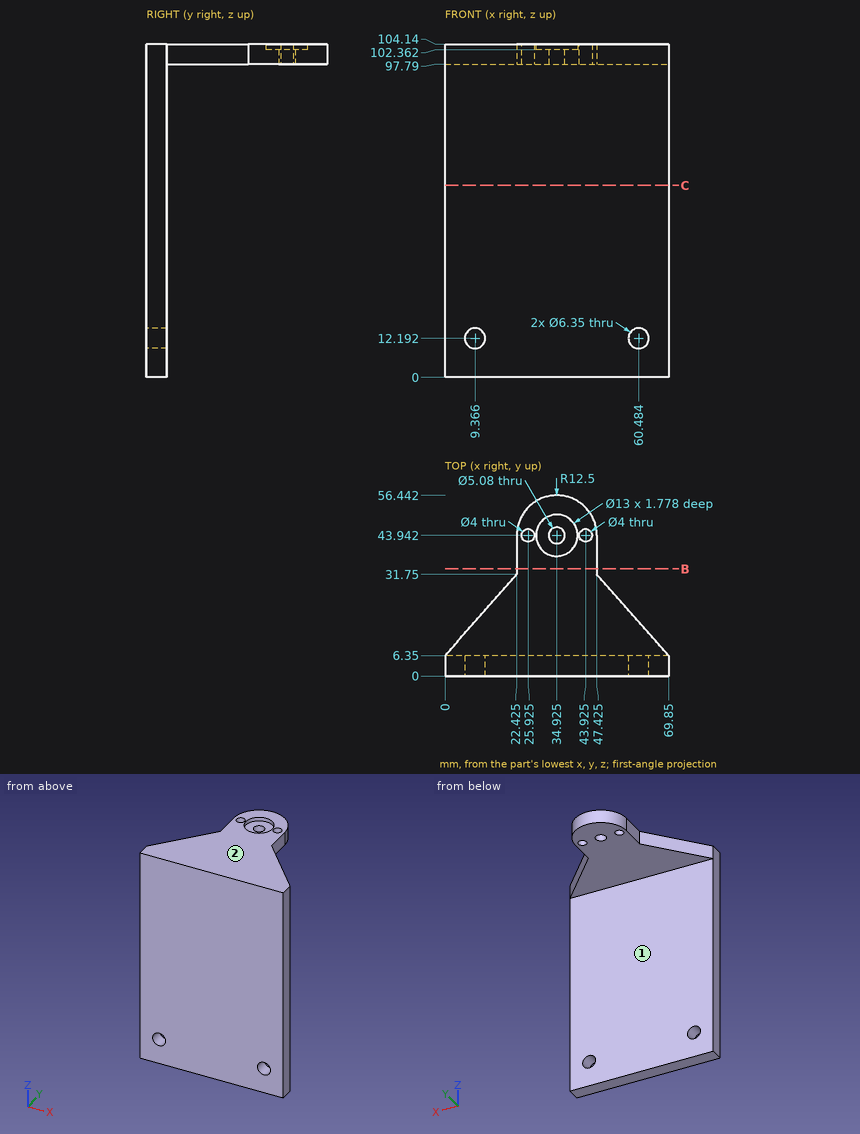
Drawing for the job (mm, zero at the part's lowest x, y, z). A direction names the side the tool comes from. Give positions to 0.01 mm unless a question says otherwise; leave off trailing zeros. Order: outer loops, then holes, each group sorted by start corner. A loop starts at its lowest first (then second) coordinate and runs counter-clockwise, first axis right, second up. Notation, with made-up numbers: M 38,83.5 L 94,83.5 A19 cw 94,95.5 Z; hole C 39.5,77.25 d8. An arc over 180 degrees is marked long. Put each result on its own line as item: value.
Item 1: 3-axis set-ups, long thin cutter, end or side, ignore diameter. For the marked faces 1 and 2: which of +Z, -Z, +X, -X, +Y, -Y reach the whole face in a straight line?
From the geometry:
face 1: -Z, +X, -X, +Y
face 2: +Z, +X, -X, +Y, -Y
Item 2: Flat gauge pins, fed straight in: pin 1 Ø5 at (x, z) = (27.5, 69) entering from +Y; pin 2 Ø15 at (x, y) = (28, 26) entering from -Z; pin 3 Ø3 at (x, y) = (25.925, 43.942) entering from +Z; pin 4 Ø3 at (y, z) = (38.5, 100.5) entering from +X (3 decimals). Where does each tip first touch, or does it go through?
From the geometry:
pin 1: stops at y = 6.35
pin 2: stops at z = 97.79
pin 3: passes through
pin 4: stops at x = 47.425
Item 3: Slice it at C-C, the plane z = 60. Write the cut outline in (x, y).
From the geometry:
outline: M 0,0 L 69.85,0 L 69.85,6.35 L 0,6.35 Z
Item 4: Slice it at B-B, the plane y = 33.5. Write the cut outline in (x, z) (3 decimals), plus the area to 3 significant figures.
From the geometry:
outline: M 22.425,97.79 L 47.425,97.79 L 47.425,104.14 L 22.425,104.14 Z
area: 159 mm2
Item 5: Probe line 1 (Y direction, x = 23, z = 82.5); line 2 (Y direction, x = 36, z = 98) (1 decimal); line 3 (Z direction, x = 8.5, y = 14). List the from-to ranges inside material, lowest first. Write a range as [from, to].
From the geometry:
line 1: y = [0, 6.35]
line 2: y = [0, 41.6], [46.2, 56.4]
line 3: z = [97.79, 104.14]
